For this review, take the finished solid that the model builds, in its own axes (mm). A direction names the side the tool comes from. Coordinates: 2 decimals unless noted, no trailing zeros. Write each loop counter-clockwise with the first axis right and the second up, starting at its lowest first coordinate (ties: lowest second). Pieces come first, ordered by that corner, then holes.
1) We need section A-A on z = 9.5. Write out the cut boundary in (x, y).
2) To check wall thickness, follow line 1 along Y through (x, z) = (-3, 7.95); line 2 along X through (y, z) = (8, 6.25); line 3 along Y through (x, z) = (-9, 9.75). State the ranges of each line that lie inside material, in increasing order.
3) For faces 5 (the face through (-9.25, 0, 9)), 6 (the face through (-16, 0, 8.3)), 7 (the face through (-9.5, 7, 3)), list the 3-axis set-ups (+Z, -Z, +X, -X, +Y, -Y) from which the entire face can be reached by the end or side of a thin tool; tool diameter is ignored.
4) Mouldability with a two-part tool opening along X and no side actions: class faces 1 (the face through (-18, -2, 5)), 2 (the face through (9.753, -0.166, 4.092)), 3 (the face through (2, 0, 6.4)), 4 (the face through (-14, -6, 0)) as pulls with the +X half, pulls with the -X half, needs draft (parallel to the pull), parting line crosses it, or undercut.
5) We need section D-D on z = 4.75. Write out the cut boundary in (x, y).
6) Insertion check: P1, Ø3, axis at x = -3, y = 6.5, coming from the -Z side; P2, Ø5, axis at x = -1, z = 3.5, coming from the +Y side; P3, Ø5, axis at x = -14, y = 0, coming from the -Z side. Each pin has a flat end and moves straight along its axis. Give the tip position at first contact, or say it passes through.
7) We need section C-C on y = 0. Write out the cut boundary in (x, z).
8) We need section B-B on x = -14. Write out the cut boundary in (y, z), then the cut area to 3 significant figures.
Autodesk Fusion 360 part; units mm, degrees
sketch "Skizze1" plane through (0, 0, 0) normal (0, 0, 1) x (1, 0, 0)
  line L0 (18, -9) -> (-18, -9)
  line L1 (-18, -9) -> (-18, 9)
  line L2 (-18, 9) -> (18, 9)
  line L3 (18, 9) -> (18, -9)
  line L4 (18, -9) -> (-18, 9) construction
  line L5 (-18, -9) -> (18, 9) construction
  line L6 (-14, 14.295) -> (-14, -12) construction
  line L7 (14, 15.3346) -> (14, -11.7486) construction
  line L8 (-3, 14) -> (-3, -10) construction
  line L9 (-21.8783, 0) -> (29.3882, 0) construction
  circle A0 centre (-3, 0) radius 3.65
  circle A1 centre (-14, 0) radius 1.75
  circle A2 centre (14, 0) radius 1.75
  line L10 (-9.5, 9) -> (-9.5, -9)
  line L11 (9.5, 9) -> (9.5, -9)
  circle A3 centre (-3, 0) radius 7.75
  line L12 (3, -6.25) -> (-9, -6.25)
  line L13 (-9, -6.25) -> (-9, 6.25)
  line L14 (-9, 6.25) -> (3, 6.25)
  line L15 (3, 6.25) -> (3, -6.25)
  line L16 (3, -6.25) -> (-9, 6.25) construction
  line L17 (-9, -6.25) -> (3, 6.25) construction
  circle A4 centre (-14, 0) radius 4.25
  circle A5 centre (14, 0) radius 4.25
  point P0 (-6.65, 0)
  point P1 (-3, 0)
  dimension "d1" = 36
  dimension "d2" = 18
  dimension "d3" = 4
  dimension "d4" = 11
  dimension "d5" = 17
  dimension "d6" = 7.3
  dimension "d7" = 3.5
  dimension "d8" = 3.5
  dimension "d10" = 4.5
  dimension "d11" = 2.85
  dimension "d12" = 15.5
  dimension "d13" = 4.5
  dimension "d14" = 12
  dimension "d15" = 12.5
  dimension "d16" = 8.5
  dimension "d17" = 8.5
extrude "Extrusion1" add sketch "Skizze1" along normal blind 10.3 contours L0 L2 L3 L11 A5 | L0 L2 L10 L11 A3 L12 L13 L14 L15 | L3 A5 | L0 L1 L10 A3 A4 | L10 A3 A4 | L10 A3 L13 | L1 L2 L10 A3 A4 | L1 A3 A4 | A3 A4 | A3 L12 L13 L14 L15 | A3 L12 L13 | A3 L13 L14 | A3 L12 | A3 L14 | A3 L12 L15 | A3 L14 L15 | A3 L15 picked at (17.25, 0)
extrude "Extrusion2" cut sketch "Skizze1" along normal blind 8.3 contours L3 A5 | L1 A3 A4 | A3 A4 picked at (17.25, 0)
extrude "Extrusion3" cut sketch "Skizze1" along normal blind 6.4 contours L10 A3 A4 | L10 A3 L13 | A3 L12 L13 L14 L15 | A3 L12 | A3 L14 | A3 L15
extrude "Extrusion4" cut sketch "Skizze1" along normal blind 6.4 contours L0 L2 L10 L11 A3 L12 L13 L14 L15 | A3 L12 L13 | A3 L13 L14 | A3 L12 L15 | A3 L14 L15
sketch "Skizze2" plane through (0, 0, 10.3) normal (0, 0, 1) x (-1, 0, 0)
  circle A0 centre (-14, 0) radius 1.75
  circle A1 centre (14, 0) radius 1.75
  circle A2 centre (3, 0) radius 3.65
  line L0 (-18, -9) -> (18, -9)
  line L1 (18, -9) -> (18, 9)
  line L2 (18, 9) -> (-18, 9)
  line L3 (-18, 9) -> (-18, -9)
  line L4 (19.6534, 0) -> (-19.2741, 0) construction
  line L5 (3, -11.2204) -> (3, 11) construction
  line L6 (-3.25, 6.5) -> (9.25, 6.5)
  line L7 (9.25, 6.5) -> (9.25, -6.5)
  line L8 (9.25, -6.5) -> (-3.25, -6.5)
  line L9 (-3.25, -6.5) -> (-3.25, 6.5)
  line L10 (-3.25, 6.5) -> (9.25, -6.5) construction
  line L11 (9.25, 6.5) -> (-3.25, -6.5) construction
  circle A3 centre (3, -6.5) radius 1.25
  point P0 (3, 0)
  point P1 (3, 0)
  point P2 (3, -6.5)
  dimension "d26" = 13
  dimension "d27" = 12.5
  dimension "d30" = 2.5
extrude "Extrusion5" cut sketch "Skizze2" against normal blind 1.92 contours L6 L7 L8 L9 A3 | L8 A3 picked at (3.3396, -6.2032)
extrude "Extrusion6" cut sketch "Skizze2" against normal blind 9 contours L8 A3 | L8 A3
Result:
1. outline: (-18, -9) - (18, -9) - (18, 9) - (-18, 9) - close; hole circle Ø3.5 at (-14, 0); hole (-9.25, -6.5) - (3.25, -6.5) - (3.25, 6.5) - (-1.75, 6.5) arc R1.25 ccw to (-4.25, 6.5) - (-9.25, 6.5) - close; hole circle Ø3.5 at (14, 0)
2. line 1: y = -9 to -3.65, 3.65 to 5.25, 7.75 to 9
2. line 2: x = -18 to -9.5, 9.5 to 18
2. line 3: y = -9 to -6.5, 6.5 to 9
3. face 5: +Z
3. face 6: -Z
3. face 7: -Z, +Y, -Y
4. face 1: pulls with the -X half
4. face 2: undercut
4. face 3: undercut
4. face 4: needs draft
5. outline: (-18, -9) - (-9.5, -9) - (-9.5, -4.22) arc R7.75 cw to (-10.41, -2.27) arc R4.25 cw to (-18, -1.44) - close; (-18, 1.44) arc R4.25 cw to (-10.41, 2.27) arc R7.75 cw to (-9.5, 4.22) - (-9.5, 9) - (-18, 9) - close; (9.5, -9) - (18, -9) - (18, -1.44) arc R4.25 cw (long way) to (18, 1.44) - (18, 9) - (9.5, 9) - close
6. P1: stops at z = 6.4
6. P2: passes through
6. P3: stops at z = 8.3
7. outline: (-18, 8.3) - (-15.75, 8.3) - (-15.75, 10.3) - (-18, 10.3) - close; (-12.25, 8.3) - (-9.75, 8.3) - (-9.75, 6.4) - (-6.65, 6.4) - (-6.65, 8.38) - (-9.25, 8.38) - (-9.25, 10.3) - (-12.25, 10.3) - close; (0.65, 6.4) - (9.5, 6.4) - (9.5, 0) - (9.75, 0) - (9.75, 8.3) - (12.25, 8.3) - (12.25, 10.3) - (3.25, 10.3) - (3.25, 8.38) - (0.65, 8.38) - close; (15.75, 8.3) - (18, 8.3) - (18, 10.3) - (15.75, 10.3) - close
8. outline: (-9, 0) - (-4.25, 0) - (-4.25, 8.3) - (-1.75, 8.3) - (-1.75, 10.3) - (-9, 10.3) - close; (1.75, 8.3) - (4.25, 8.3) - (4.25, 0) - (9, 0) - (9, 10.3) - (1.75, 10.3) - close
8. area: 108 mm2
